For this review, take the finished solid that the model builds, in its own axes (mm). Face numbers are marked on the shaded views. Coordinates: 2 decimals unless noted, no trailing zeros. Write each loop counter-clockwise with the first axis right and the second up, starting at its lowest first coordinate (ties: lowest second). Pieces come first, ordered by that corner, then holes.
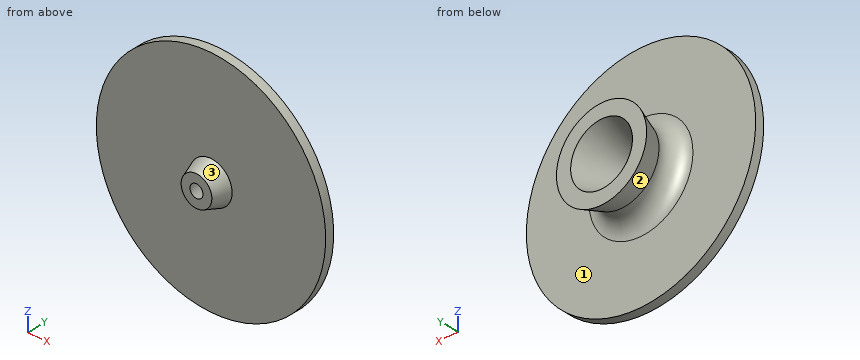
```python
from build123d import *

# Parameters (mm, degrees)
FILLET1_R = 10


with BuildPart() as part:
    # Sketch1 → Revolve1 (revolve)
    with BuildSketch(Plane.XY, mode=Mode.PRIVATE) as revolve1_sk:
        Polygon((-18.744174885, 0), (-72.691581878, 0), (-72.691581878, -5.616084741), (-13.370797043, -5.616084741), (-9.742614484, -15.774995906), (-4.108687375, -15.774995906), (-9.742614484, 0), (-19.607603388, 27.621968933), (-28.609163789, 27.621968933), align=None)
    revolve(revolve1_sk.sketch.rotate(Axis((0, 0, 0), (0, 1, 0)), 270), axis=Axis((0, 0, 0), (0, 1, 0)))

    # Fillet1
    fillet1_edges = [part.edges().sort_by_distance(p)[0] for p in [
        (0, 0, 18.744174885),
    ]]
    fillet(fillet1_edges, radius=FILLET1_R)


solid = part.part
```
Q1. Add section A-A (y = 21). State the section outline as (x, z) points.
Ans:
outline: circle Ø52.49 at (0, 0); hole circle Ø34.49 at (0, 0)
Q2. For probe 1 along Y at (x, z) = (53, 6.5); probe 2 along Z at (x, y) = (6, 13.5); probe 3 along Z at (x, y) = (5, 4), list the stretches that pass through material, from the lowest coordinate up.
Ans:
probe 1: y = -5.62 to 0
probe 2: z = -22.79 to -13.27, 13.27 to 22.79
probe 3: z = -24.43 to -9.99, 9.99 to 24.43
Q3. Clearance check with flat-ended pins moving along their axes: pin 1 Ø12 at (y, z) = (-5.5, -44) entering from -X; pin 2 Ø12 at (y, z) = (4.5, 8) entering from -X; pin 3 Ø5 at (y, z) = (16, 14) entering from -X. State where each tip first meets the part, or that it passes through.
Ans:
pin 1: stops at x = -61.97
pin 2: stops at x = -72.58
pin 3: stops at x = -21.93
Q4. Add section C-C (x = -61). State the section outline as (y, z) points, then the cut area to 3 significant figures.
Ans:
outline: (-5.62, -39.54) - (0, -39.54) - (0, 39.54) - (-5.62, 39.54) - close
area: 444 mm2
Q5. Add section D-D (y = -9). State the section outline as (x, z) points, then the cut area to 3 significant figures.
Ans:
outline: circle Ø24.32 at (0, 0); hole circle Ø13.06 at (0, 0)
area: 331 mm2
Q6. Draft analysis for pull direction Y (two halves, no side actions). For the marked faces 1, 2 and 3, state which applies: +Y half, -Y half, draft (parallel to the pull), parting line (faces both ways), or undercut.
Ans:
face 1: +Y half
face 2: undercut
face 3: -Y half
Q7. Add section B-B (z = 52). State the section outline as (x, y) points.
Ans:
outline: (-50.79, -5.62) - (50.79, -5.62) - (50.79, 0) - (-50.79, 0) - close
